Print and shaded views of the part. All mm, measured from the part's lowest x, y and z. Round coordinates to 2 decimals unless told otherwise and drop trailing zeros. Order: outer loops, then holes, each group sorted by start corner. A loop starts at its lowest first (then second) coordinate and runs counter-clockwise, first axis right, second up. Notation, with made-up numbers: (77, -39) - (117, -39) arc R28 ccw to (117, -20) - close; hole circle Ø5 at (60, 41.5). An arc over 180 degrees is marked (long way). Return JSON: item names as keys, results as strings. Group by question number.
Item 1: Saw through at B-B on y = 3.5. List the corners of the cut face in (x, z), and give its area (4 significant figures).
Item 2: Probe probe 1 along Y at (x, z) = (47, 4.45); probe 2 along Y at (x, z) = (2.5, 1.75); probe 3 along Y at (x, z) = (15, 2.95). List the from-to ranges inside material, lowest first.
Item 3: Saw through at C-C on x = 10. List the corners of the cut face in (y, z).
Item 4: Saw through at D-D on z = 2.65. List the corners of the cut face in (x, y).
Item 5: Saw through at A-A on x = 47. List the corners of the cut face in (y, z), and give its area (3 significant figures).
Item 6: Drop flat-ended pins along their axis: pin 1 (2.5 mm diameter, centred on x = 47, y = 28, fed in from -Z); pin 2 (4 mm diameter, centred on x = 47, y = 3.5, fed in from -Z); pin 3 (3 mm diameter, centred on x = 15.5, y = 21, fed in from +Z). Give the stop position or say it passes through.
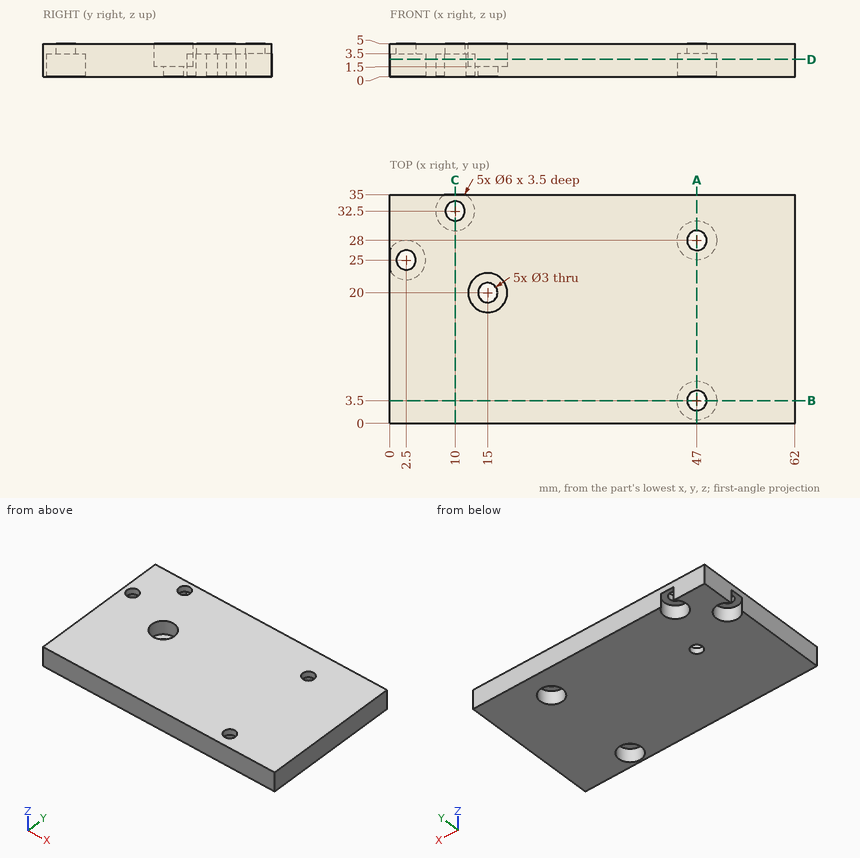
Filled in:
{
 "1": {"outline": "(0, 0) - (44, 0) - (44, 3.5) - (45.5, 3.5) - (45.5, 5) - (0, 5) - close; (48.5, 3.5) - (50, 3.5) - (50, 0) - (62, 0) - (62, 5) - (48.5, 5) - close", "area": "284.5 mm^2"},
 "2": {"probe 1": "y = 0 to 2, 5 to 26.5, 29.5 to 35", "probe 2": "y = 0 to 22, 28 to 35", "probe 3": "y = 0 to 17, 23 to 35"},
 "3": {"outline": "(0, 0) - (29.5, 0) - (29.5, 3.5) - (31, 3.5) - (31, 5) - (0, 5) - close; (34, 3.5) - (35, 3.5) - (35, 5) - (34, 5) - close"},
 "4": {"outline": "(0, 0) - (62, 0) - (62, 35) - (11.66, 35) arc R3 cw (long way) to (8.34, 35) - (0, 35) - (0, 26.66) arc R3 cw (long way) to (0, 23.34) - close; hole circle Ø6 at (15, 20); hole circle Ø6 at (47, 3.5); hole circle Ø6 at (47, 28)"},
 "5": {"outline": "(0, 0) - (0.5, 0) - (0.5, 3.5) - (2, 3.5) - (2, 5) - (0, 5) - close; (5, 3.5) - (6.5, 3.5) - (6.5, 0) - (25, 0) - (25, 3.5) - (26.5, 3.5) - (26.5, 5) - (5, 5) - close; (29.5, 3.5) - (31, 3.5) - (31, 0) - (35, 0) - (35, 5) - (29.5, 5) - close", "area": "124 mm^2"},
 "6": {"pin 1": "passes through", "pin 2": "stops at z = 3.5", "pin 3": "stops at z = 1.5"}
}
